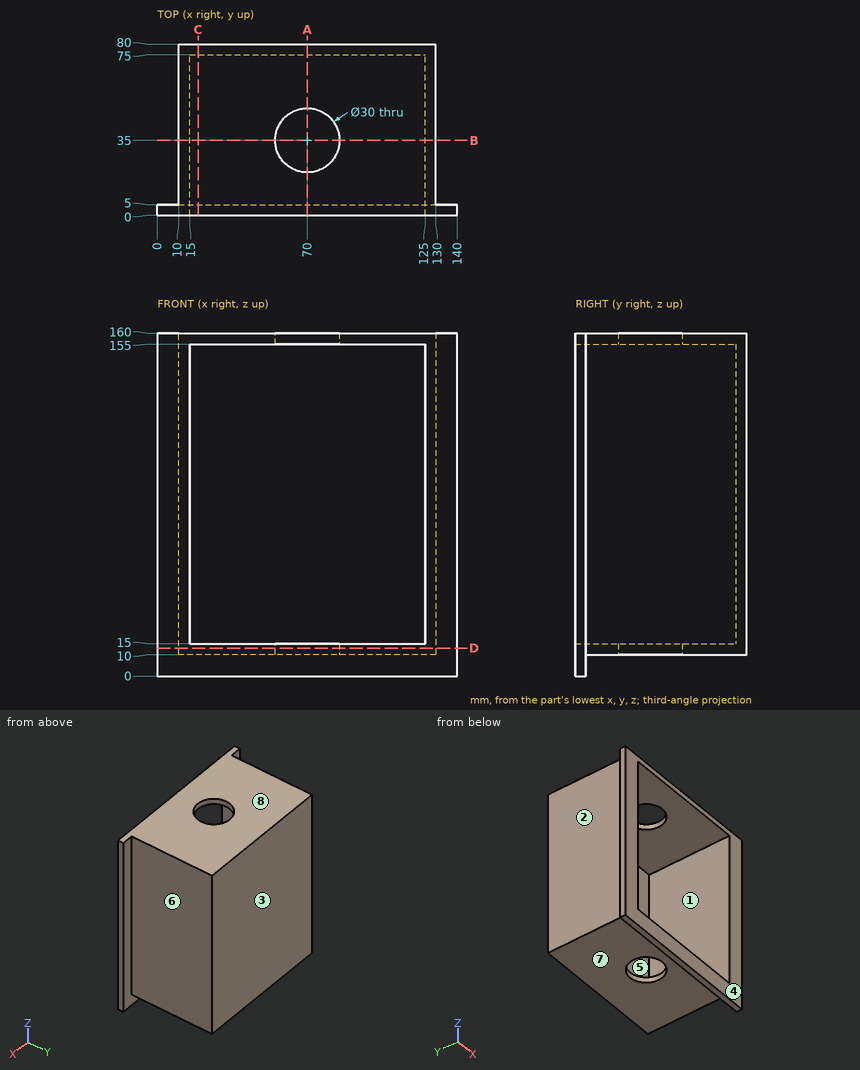
Here's the drawing with two shaded views (mm, measured from the low corner). I have some questions. A direction names the side the tool comes from. Coordinates: 2 decimals unless noted, no trailing zeros. Write each loop counter-clockwise with the first axis right and the second up, starting at its lowest first coordinate (ties: lowest second). Pieces come first, ordered by that corner, then holes. Notation, with made-up numbers: (-9, 17) -> (27, 17) arc R35 cw to (27, 56) -> close; hole circle Ø11 at (35, 73). An arc over 180 degrees is marked (long way). Answer as CSV lines item,"result".
1) If we mould it in two halves opening along X, with no side actions, what happens to the marked faces 1, 2 and 3? For each: +X half, -X half, draft (parallel to the pull), parting line (faces both ways), or undercut.
Check result:
face 1,"undercut"
face 2,"-X half"
face 3,"draft"
2) If we section it at B-B on y = 35: Please give me the cut outline in (x, z).
Check result:
outline,"(10, 10) -> (55, 10) -> (55, 15) -> (15, 15) -> (15, 155) -> (55, 155) -> (55, 160) -> (10, 160) -> close; (85, 10) -> (130, 10) -> (130, 160) -> (85, 160) -> (85, 155) -> (125, 155) -> (125, 15) -> (85, 15) -> close"
3) Will these pins go through, and if not, where does the flat tip stop? P1, Ø10, axis at y = 52, z = 29.5, coming from the -X side; P2, Ø12, axis at x = 19, y = 29, coming from the -Z side; P3, Ø8, axis at x = 84, z = 34.5, coming from the -Y side.
Check result:
P1,"x = 10"
P2,"z = 10"
P3,"y = 75"
4) If we section it at A-A on x = 70: Please give me the cut outline in (y, z), then the cut area to 3 significant figures.
Check result:
outline,"(0, 0) -> (5, 0) -> (5, 10) -> (20, 10) -> (20, 15) -> (0, 15) -> close; (0, 155) -> (20, 155) -> (20, 160) -> (0, 160) -> close; (50, 10) -> (80, 10) -> (80, 160) -> (50, 160) -> (50, 155) -> (75, 155) -> (75, 15) -> (50, 15) -> close"
area,"1,250 mm²"
5) On a 3-axis mill with a long thin cutter (end or side, diameter ignored), from which of +Z, -Z, +X, -X, +Y, -Y can I reach the whole of each face in a straight line? I mean the marked faces 4, 5, 6, 7 and 8. Say none if no direction works.
Check result:
face 4,"+Z, -Z, +X, -X, -Y"
face 5,"-Y"
face 6,"+Z, -Z, +X, +Y"
face 7,"-Z, +X, -X, +Y"
face 8,"+Z, +X, -X, +Y, -Y"
6) If we section it at D-D on z = 13: Please give me the cut outline in (x, y), then the cut area to 3 significant figures.
Check result:
outline,"(0, 0) -> (140, 0) -> (140, 5) -> (130, 5) -> (130, 80) -> (10, 80) -> (10, 5) -> (0, 5) -> close; hole circle Ø30 at (70, 35)"
area,"8,990 mm²"
7) If we section it at C-C on x = 19: Please give me the cut outline in (y, z).
Check result:
outline,"(0, 0) -> (5, 0) -> (5, 10) -> (80, 10) -> (80, 160) -> (0, 160) -> (0, 155) -> (75, 155) -> (75, 15) -> (0, 15) -> close"
8) If I drill on line 1 (X direction, y = 38, z = 132); line 2 (Z direction, x = 85, y = 73); line 3 (Y direction, x = 70, z = 13.75), over which ranges is the centre line in solid material (lowest first)? Write a range as from..to.
Check result:
line 1,"10..15, 125..130"
line 2,"10..15, 155..160"
line 3,"0..20, 50..80"
